```python
from build123d import *

# Parameters (mm, degrees)
F0_W     = 800
F0_H     = 27
F1_DEPTH = 2000
F2_R     = 50.336574
F3_DEPTH = 700


with BuildPart() as f1:
    # F0 (on Front) → F1 (new body)
    with BuildSketch(Plane.XZ):
        with Locations((0, 713.5)):
            Rectangle(F0_W, F0_H)
    extrude(amount=F1_DEPTH)

    # F2 (on face) → F3 (join)
    with BuildSketch(Plane(origin=(0, 0, 700), x_dir=(1, 0, 0), z_dir=(0, 0, -1))):
        with Locations((-250, 400)):
            Circle(F2_R)
        with Locations((-250, 1600)):
            Circle(F2_R)
        with Locations((250, 1600)):
            Circle(F2_R)
        with Locations((250, 400)):
            Circle(F2_R)
    extrude(amount=F3_DEPTH)


solid = f1.part
```
For this review, take the finished solid that the model builds, in its own axes (mm). A direction names the side the tool comes from. Coordinates: 2 decimals unless noted, no trailing zeros. Write each loop counter-clockwise with the first axis right and the second up, starting at its lowest first coordinate (ties: lowest second). Pieces come first, ordered by that corner, then holes.
(1) For pin 1 Ø5 at (x, y) = (-171.5, -1158.5) entering from -Z; pin 2 Ø4 at (x, z) = (-256, 267) entering from +Y; pin 3 Ø1 at (x, z) = (-271.5, 594) entering from -Y, all flat-tipped, find the tip position at first contact; note any pin that passes through.
(2) Add section B-B on x = 250. Give the boundary of the cut face in (y, z).
(3) The part is to be moulded in two halves that separate along X. For faces 1 (the face through (239.09, -1550.86, 354.9)), 2 (the face through (-260.91, -1550.86, 354.9)), 3 (the face through (-6, -986, 727)), say which applies: +X half, -X half, draft (parallel to the pull), parting line (faces both ways), or undercut.
(4) Add section D-D on x = 128. Give the boundary of the cut face in (y, z), then the cut area to 3 significant figures.
(5) Tool access review of faces 4 (the face through (-222.939, -442.444, 354.9)), 5 (the face through (-251, -1601, 0)): name each direction out of +Z, -Z, +X, -X, +Y, -Y from which nothing blocks a thin tool from reaching the whole face with its end or side.
(6) Wall thickness on probe 1 along Y at (x, z) = (-252, 591); probe 2 along Z at (x, y) = (263, -1913.5); probe 3 along Y at (x, z) = (-208, 148): over which ranges is each line inside the solid? List them lowest first.
(7) Add section C-C on z = 505.5. Give the boundary of the cut face in (x, y), then the cut area to 3 significant figures.
(8) Add section A-A on y = -400. Give the boundary of the cut face in (x, z).
Answer sheet:
1. pin 1: stops at z = 700
1. pin 2: stops at y = -349.82
1. pin 3: stops at y = -1645.75
2. outline: (-2000, 700) - (-1650.34, 700) - (-1650.34, 0) - (-1549.66, 0) - (-1549.66, 700) - (-450.34, 700) - (-450.34, 0) - (-349.66, 0) - (-349.66, 700) - (0, 700) - (0, 727) - (-2000, 727) - close
3. face 1: undercut
3. face 2: undercut
3. face 3: draft
4. outline: (-2000, 700) - (0, 700) - (0, 727) - (-2000, 727) - close
4. area: 54,000 mm2
5. face 4: -Z
5. face 5: -Z, +X, -X, +Y, -Y
6. probe 1: y = -1650.3 to -1549.7, -450.3 to -349.7
6. probe 2: z = 700 to 727
6. probe 3: y = -1627.74 to -1572.26, -427.74 to -372.26
7. outline: circle Ø100.67 at (-250, -1600); circle Ø100.67 at (-250, -400); circle Ø100.67 at (250, -1600); circle Ø100.67 at (250, -400)
7. area: 31,800 mm2
8. outline: (-400, 700) - (-300.34, 700) - (-300.34, 0) - (-199.66, 0) - (-199.66, 700) - (199.66, 700) - (199.66, 0) - (300.34, 0) - (300.34, 700) - (400, 700) - (400, 727) - (-400, 727) - close
